Part print with two shaded views. Sizes in mm from the minimum x, y, z corner. A direction names the side the tool comes from. Give positions to 0.01 mm unless a question says otherwise; leave off trailing zeros. Loops run counter-clockwise (first coordinate to the right, second up) from the corner with the lowest first, then second, coordinate; pieces in that order, holes last. Notation, with made-up numbers: (43.25, 7.25) -> (47.25, 7.25) arc R29 cw to (47.25, 33.25) -> close; hole circle Ø3 at (80, 86). An arc over 180 degrees is marked (long way). One line per question, with ' | ' between items. Start each with the question number.
(1) 3-axis set-ups, long thin cutter, end or side, ignore diameter. For the marked faces 4, 5 and 6: which of +Z, -Z, +X, -X, +Y, -Y reach the whole face in a straight line?
(2) Slice it at D-D, the plane y = 6.75. Write the cut outline in (x, z) (1 decimal).
(3) Drill centre lines: L1, parallel to Z at x = 1.35, y = 2.5; L2, parallel to X at y = 5, z = 2.75; L3, parallel to X at y = 2, z = 2.75. Where is each one in solid material? Low to high. Write a range as from..to.
(4) Slice it at B-B, the plane z = 3.25. Write the cut outline in (x, y).
(5) Slice it at C-C, the plane y = 5.5. Write the cut outline in (x, z), then the cut area to 3 significant figures.
(6) Flat gauge pin, fed straight in: pin 1 Ø1.5 at (y, z) = (2, 4) entering from -X. Where does the tip first touch, or does it go through?
(7) Mould opens along Y. For the marked faces 1, 2 and 3 say: pulls with the +Y half, pulls with the -Y half, needs draft (parallel to the pull), parting line crosses it, or undercut.
(8) Slice it at A-A, the plane x = 0.4. Write the cut outline in (y, z), then the cut area to 3 significant figures.
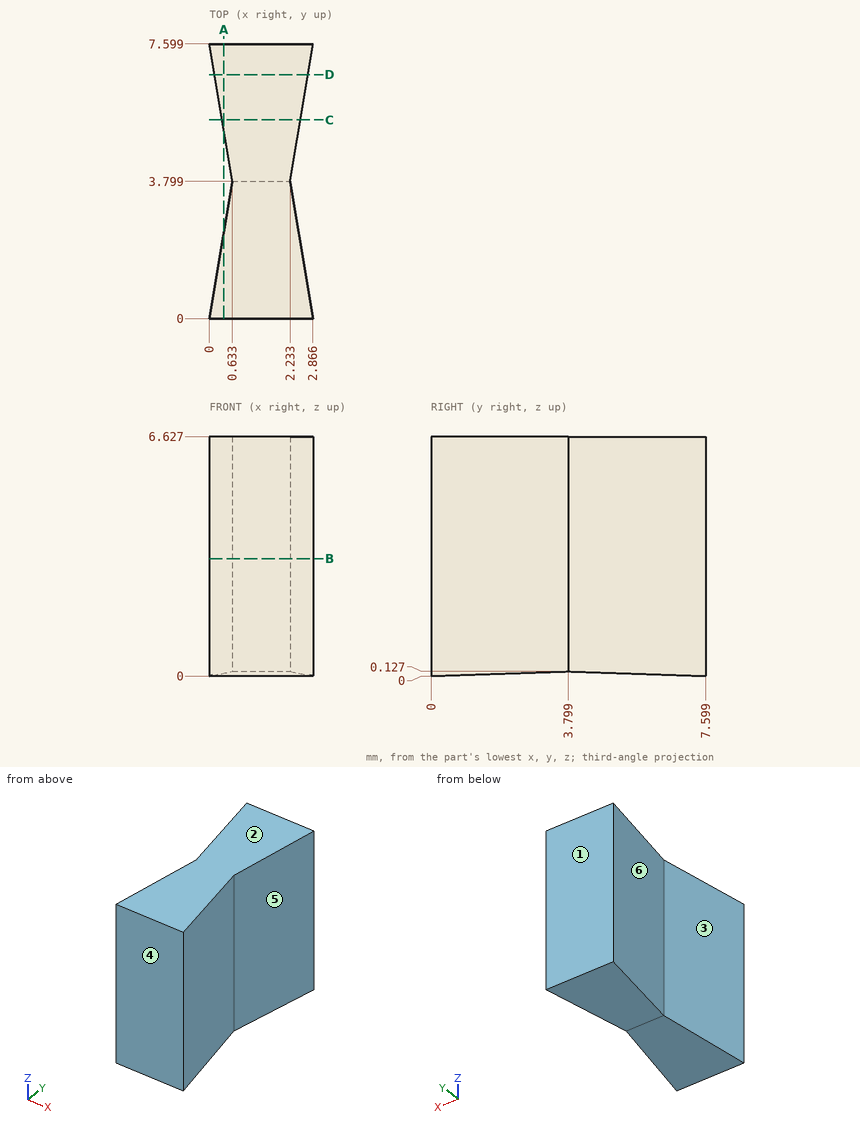
Final values:
1) face 4: +Z, -Z, +X, -X, -Y | face 5: +Z, -Z, +X | face 6: +Z, -Z, -X
2) outline: (0.1, 0) -> (2.7, 0) -> (2.7, 6.6) -> (0.1, 6.6) -> close
3) L1: 0.08..6.63 | L2: 0.43..2.43 | L3: 0.33..2.53
4) outline: (0, 0) -> (2.87, 0) -> (2.23, 3.8) -> (2.87, 7.6) -> (0, 7.6) -> (0.63, 3.8) -> close
5) outline: (0.35, 0.07) -> (2.52, 0.07) -> (2.52, 6.63) -> (0.35, 6.63) -> close | area: 14.2 mm2
6) pin 1: x = 0.21
7) face 1: pulls with the +Y half | face 2: needs draft | face 3: undercut
8) outline: (0, 0) -> (2.4, 0.08) -> (2.4, 6.63) -> (0, 6.63) -> close; (5.2, 0.08) -> (7.6, 0) -> (7.6, 6.63) -> (5.2, 6.63) -> close | area: 31.6 mm2
